Here's how the part is built. I have some questions about the finished solid (model axes, mm). Face numbers are marked on the shaded views. Give positions to 0.01 mm unless a question says otherwise; leave off trailing zeros. Loops run counter-clockwise (first coordinate to the right, second up) from the corner with the lowest first, then second, coordinate; pieces in that order, holes last. Notation, with made-up numbers: M 72.25,-37.75 L 120.25,-37.75 A36 cw 120.25,1.25 Z; hole C 57.25,29 d5. An arc over 180 degrees is marked long. Write item = value, one per line. Start each with the question number.
```python
from build123d import *

# Parameters (mm, degrees)
F0_W     = 710
F0_H     = 35
F1_DEPTH = 2050
F2_W     = 500
F2_H     = 350
F2_H_2   = 1080
F3_DEPTH = 10


with BuildPart() as f1:
    # F0 (on Top) → F1 (new body)
    with BuildSketch(Plane.XY):
        with Locations((0, 17.5)):
            Rectangle(F0_W, F0_H)
    extrude(amount=F1_DEPTH)

    # F2 (on face) → F3 (cut)
    with BuildSketch(Plane.XZ):
        with Locations((5, 425)):
            Rectangle(F2_W, F2_H)
        with Locations((5, 1390)):
            Rectangle(F2_W, F2_H_2)
    extrude(amount=-F3_DEPTH, mode=Mode.SUBTRACT)

    # F6: sweep along a path in F5
    with BuildLine(Plane.XZ.offset(-10)) as f6_path:
        Line((255, 1930), (-245, 1930))
        Line((-245, 1930), (-245, 850))
        Line((-245, 850), (255, 850))
        Line((255, 850), (255, 1930))
    # F4 (on Right) → F6 (sweep)
    with BuildSketch(Plane.YZ):
        with BuildLine():
            Line((-10, 850), (10, 850))
            Line((10, 850), (10, 860.4986502942))
            Line((10, 860.4986502942), (-2, 860.4986502942))
            Line((-2, 860.4986502942), (-2, 857.4986502942))
            Line((-2, 857.4986502942), (-5.9265357135, 857.4986502942))
            Line((-5.9265357135, 857.4986502942), (-5.9265357135, 854.9986502942))
            ThreePointArc((-5.9265357135, 854.9986502942), (-7.387997015, 854.4399528765), (-8, 853))
            Line((-8, 853), (-10, 853))
            Line((-10, 853), (-10, 850))
        make_face()
    sweep(path=f6_path.line, transition=Transition.RIGHT)

    # F9: sweep along a path in F8
    with BuildLine(Plane.XZ.offset(-10)) as f9_path:
        Line((255, 600), (-245, 600))
        Line((-245, 600), (-245, 250))
        Line((-245, 250), (255, 250))
        Line((255, 250), (255, 600))
    # F7 (on Right) → F9 (sweep)
    with BuildSketch(Plane.YZ):
        with BuildLine():
            Line((-10, 250), (10, 250))
            Line((10, 250), (10, 260.4986502942))
            Line((10, 260.4986502942), (-2, 260.4986502942))
            Line((-2, 260.4986502942), (-2, 257.4986502942))
            Line((-2, 257.4986502942), (-5.9265357135, 257.4986502942))
            Line((-5.9265357135, 257.4986502942), (-5.9265357135, 254.9986502942))
            ThreePointArc((-5.9265357135, 254.9986502942), (-7.387997015, 254.4399528765), (-8, 253))
            Line((-8, 253), (-10, 253))
            Line((-10, 253), (-10, 250))
        make_face()
    sweep(path=f9_path.line, transition=Transition.RIGHT)


solid = f1.part
```
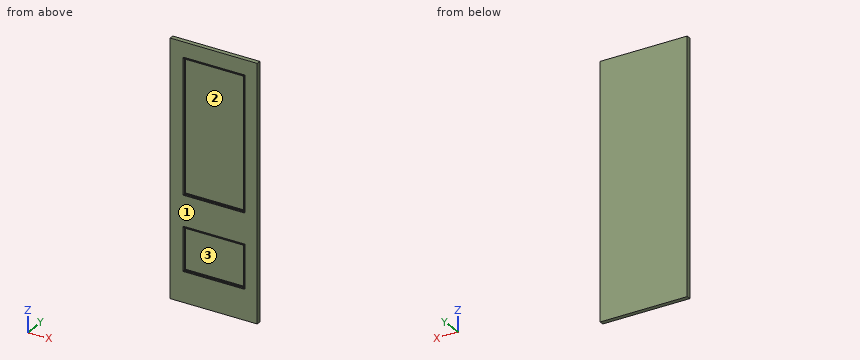
Q1. If we section it at B-B, the plane x = 287: List the corners of the cut face in (y, z) for me, then the cut area to 4 significant figures.
Q2. If we section it at C-C, the plane z = 160.5: List the corners of the cut face in (x, y) for me.
Q3. If we section it at A-A, the plane z = 1708: List the corners of the cut face in (x, y) for me.
Q4. If I drill on line 1 along Z through (x, y) = (-124.5, 6.5); line 2 along Y through (x, z) = (70, 645); line 3 along Y through (x, z) = (-117, 324.5), over which ranges is the centre line in solid material (lowest first)?
Q5. We'd pull the mould along X, two halves only. Please class the marked faces 1, 2 and 3: pulls with the +X half, pulls with the -X half, needs draft (parallel to the pull), parting line crosses it, or undercut.
Q6. Will these pins go through, and if not, where does the flat tip stop? pin 1 (3 mm diameter, centred on x = 76, y = -5, fed in from +Z); pin 2 (1.5 mm diameter, centred on x = -187, z = 523.5, fed in from -Y); pin 3 (8 mm diameter, centred on x = -75.5, y = -6.5, fed in from -Z).
Resolved:
q1.outline = M 0,0 L 35,0 L 35,2050 L 0,2050 Z
q1.area = 71,750 mm²
q2.outline = M -355,0 L 355,0 L 355,35 L -355,35 Z
q3.outline = M -355,0 L -245,0 L -245,-10 L -242,-10 L -242,-8 A2 ccw -240,-5.93 L -237.5,-5.93 L -237.5,-2 L -234.5,-2 L -234.5,10 L 244.5,10 L 244.5,-2 L 247.5,-2 L 247.5,-5.93 L 250,-5.93 A2 ccw 252,-8 L 252,-10 L 255,-10 L 255,0 L 355,0 L 355,35 L -355,35 Z
q4.line_1 = 0 to 260.5, 589.5 to 860.5, 1919.5 to 2050
q4.line_2 = 0 to 35
q4.line_3 = 10 to 35
q5.face_1 = needs draft
q5.face_2 = undercut
q5.face_3 = undercut
q6.pin_1 = 1930
q6.pin_2 = 10
q6.pin_3 = 250
